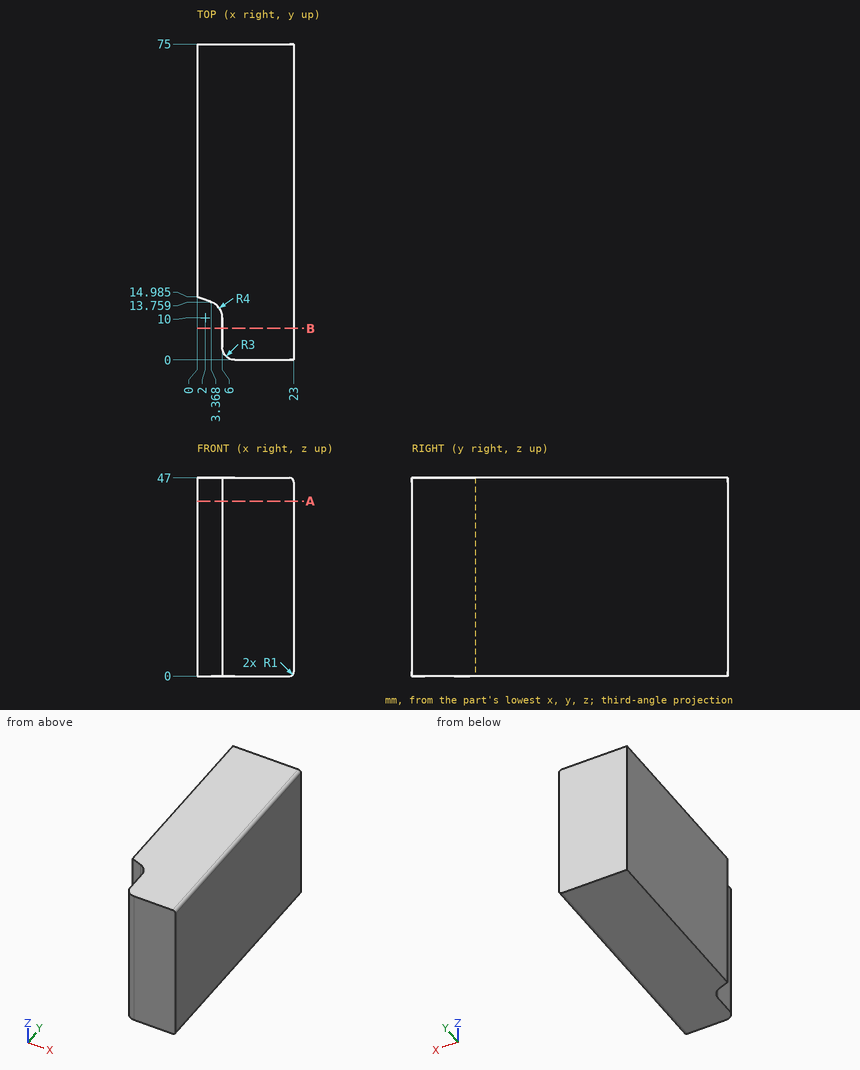
Drawing for the job (mm, zero at the part's lowest x, y, z). Coordinates: 2 decimals unless noted, no trailing zeros. Order: outer loops, then holes, each group sorted by start corner. A loop starts at its lowest first (then second) coordinate and runs counter-clockwise, first axis right, second up.
Item 1: Band-saw the part on B-B on y = 7.5. List the corners of the cut face in (x, z).
Check sheet entries:
outline: (6, 0) - (22, 0) arc R1 ccw to (23, 1) - (23, 46) arc R1 ccw to (22, 47) - (6, 47) - close
Item 2: Drill centre lines: L1, parallel to Y at x = 6.75, z = 34.5 (1 decimal); L2, parallel to Y at x = 2.25, z = 29 (1 decimal); L3, parallel to X at y = 13, z = 44 (1 decimal). Where is each one in solid material? Low to high.
Check sheet entries:
L1: y = 1 to 75
L2: y = 14.2 to 75
L3: x = 4.6 to 23
Item 3: Band-saw the part on A-A on z = 41.5. List the corners of the cut face in (x, y) (1 decimal), plus the area to 3 significant figures.
Check sheet entries:
outline: (0, 15) - (3.4, 13.8) arc R4 cw to (6, 10) - (6, 3) arc R3 ccw to (9, 0) - (23, 0) - (23, 75) - (0, 75) - close
area: 1,640 mm2
Item 4: Pin check, flat tips, straight feed: pin 1 Ø5.5 at (y, z) = (5, 32) entering from -X; pin 2 Ø2 at (y, z) = (38.5, 35) entering from -X. Stop position of each tip, or through.
Check sheet entries:
pin 1: stops at x = 6
pin 2: stops at x = 0
